Input: dimensioned drawing with shaded views. Units: mm. Origin: part minimum x, y, z. A direction names the side the tool comes from. Round coordinates to 2 decimals unless told otherwise and drop trailing zeros. Order: outer loops, then holes, each group sorted by start corner. A loop starts at its lowest first (then second) coordinate and runs counter-clockwise, first axis right, second up. Notation, with made-up numbers: M 72.25,-38 L 94.25,-38 A17 ccw 94.25,-30 Z; hole C 35,61.25 d9. An arc over 180 degrees is marked long. Use CSV: the item, a comma, the result in double quotes. Start each with the question number.
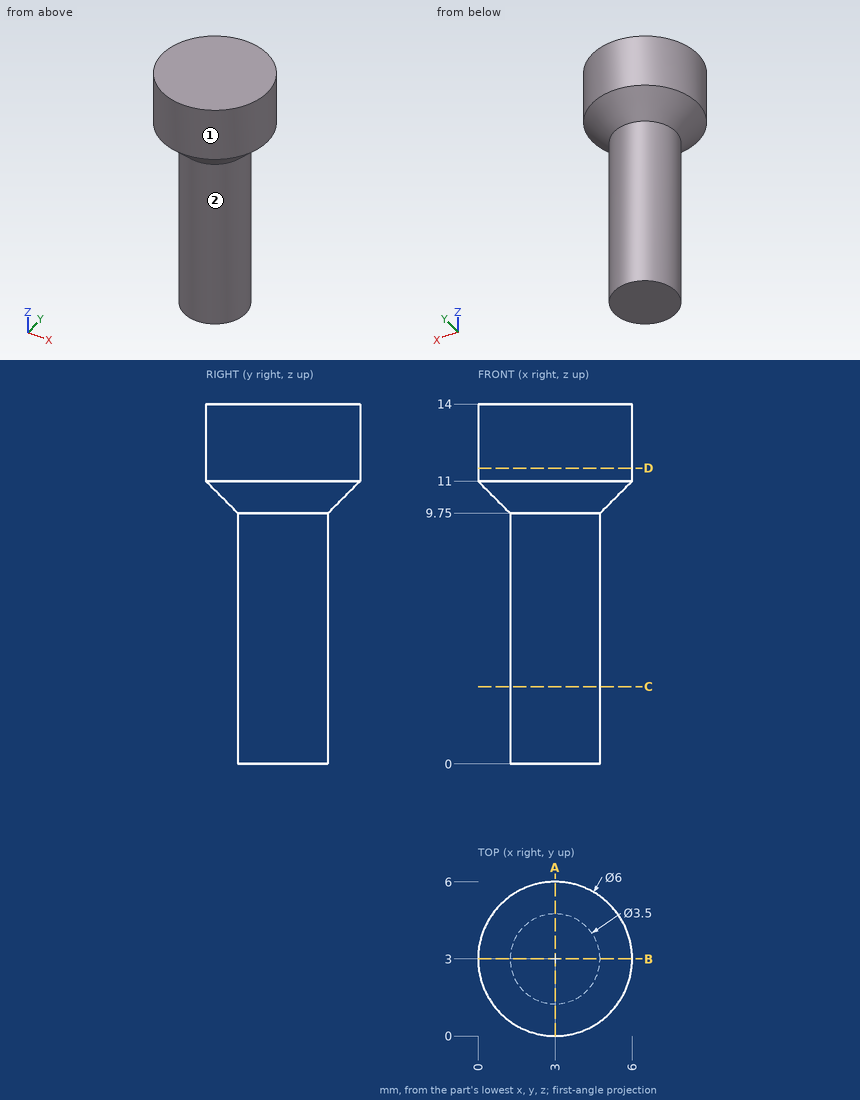
(1) Contact query for flat-ended pins moving along their axis: P1, Ø1, axis at y = 3.5, z = 1.5, coming from the -X side; P2, Ø3, axis at y = 5.5, z = 12.5, coming from the -X side. Output: stop coordinate, or through.
(2) Reachability of the marked faces 1 and 2 from +Z, -Z, +X, -X, +Y, -Y: full face, straight path, thin tool, end or side. Return the list, or none.
(3) Section C-C on z = 3. Return loops of the section in (x, y), plus the area to 3 significant figures.
(4) Section D-D on z = 11.5. Return loops of the section in (x, y), plus the area to 3 significant figures.
(5) Line query: line 1 along X through (y, z) = (2.85, 11.25); line 2 along X through (y, z) = (3.7, 10.5); line 3 along Z through (x, y) = (1.3, 5.4). Output: solid intervals per line, ascending.
(6) Section A-A on x = 3. Return loops of the section in (y, z).
Results below:
1,P1,"stops at x = 1.25"
1,P2,"stops at x = 0.17"
2,face 1,"+Z, -Z"
2,face 2,"-Z"
3,outline,"C 3,3 d3.5"
3,area,"9.62 mm2"
4,outline,"C 3,3 d6"
4,area,"28.3 mm2"
5,line 1,"x = 0 to 6"
5,line 2,"x = 0.6 to 5.4"
5,line 3,"z = 10.94 to 14"
6,outline,"M 0,11 L 1.25,9.75 L 1.25,0 L 4.75,0 L 4.75,9.75 L 6,11 L 6,14 L 0,14 Z"
